The listing builds one solid part. Answer for the finished solid, in the listing's coordinates (mm). A direction names the side the tool comes from. Round coordinates to 2 decimals unless told otherwise and drop trailing zeros. Write each loop counter-clockwise with the first axis right and the second up, starting at its lowest first coordinate (ties: lowest second). Pieces come first, ordered by that corner, then holes.
Item 1: Find section D-D on y = 30. Give the vertices of the cut face in (x, z), then the cut area to 3 significant figures.
Item 2: Each of these flat-tipped pins is pushed along its axis until it touches: pin 1 (1 mm diameter, centred on y = 10, z = 1, fed in from +X); pin 2 (0.6 mm diameter, centred on y = -1, z = 1.5, fed in from +X). Where does it stop, or does it pass through?
Item 3: Find section C-C on x = 8. Give the vertices of the cut face in (y, z), then the cut area to 3 significant figures.
Item 4: Find section B-B on y = -1. Give the vertices of the cut face in (x, z), then the cut area to 3 significant figures.
Item 5: A tool of negligible diameter and unlimited length cuts with its end or side. For faces 1 (the face through (1, 32, 1)), 2 (the face through (3.877, -2, 1)), 3 (the face through (-3.877, 22, 1)), from which of +Z, -Z, +X, -X, +Y, -Y can it reach the whole face along a straight path? Write none if from no direction.
Item 6: Find the intervals of material crossed by probe 1 along Y at (x, z) = (0.5, 0.85); probe 2 along X at (y, z) = (18.5, 0.95); probe 3 along Y at (x, z) = (3.25, 1.35), in increasing order.
Item 7: For a pull along Y with two mould halves and no side action, classify faces 4 (the face through (0, 16, 1)), 5 (the face through (2.77, 2.71, 0.99)), 6 (the face through (-2.77, -2.71, 0.99)), 7 (the face through (9, 47, 1)) as +Y half, -Y half, draft (parallel to the pull), parting line (faces both ways), or undercut.
```python
from build123d import *

# Parameters (mm, degrees)
F0_R     = 1.875
F1_DEPTH = 2
F2_R     = 4.99999


# Not quite as in the source:
# - a fillet or chamfer is up to 0.001 mm smaller than in the source, because OpenCascade refuses the exact size


with BuildPart() as f1:
    # F0 (on Top) → F1 (new body)
    with BuildSketch(Plane.XY):
        with BuildLine():
            ThreePointArc((0, 3.876953125), (-2.741419845, 2.741419845), (-3.876953125, 0))
            ThreePointArc((-3.876953125, 0), (-2.741419845, -2.741419845), (0, -3.876953125))
            ThreePointArc((0, -3.876953125), (2.741419845, -2.741419845), (3.876953125, 0))
            ThreePointArc((3.876953125, 0), (2.741419845, 2.741419845), (0, 3.876953125))
        make_face()
        Circle(F0_R, mode=Mode.SUBTRACT)
        with BuildLine():
            Line((-3.876953125, 49), (-3.876953125, 0))
            ThreePointArc((-3.876953125, 0), (-2.741419845, 2.741419845), (0, 3.876953125))
            Line((0, 3.876953125), (0, 34))
            Line((0, 34), (10, 34))
            Line((10, 34), (10, 49))
            Line((10, 49), (-3.876953125, 49))
        make_face()
        with BuildLine():
            ThreePointArc((3.876953125, 0), (2.741419845, -2.741419845), (0, -3.876953125))
            Line((0, -3.876953125), (3.876953125, -3.876953125))
            Line((3.876953125, -3.876953125), (3.876953125, 0))
        make_face()
    extrude(amount=F1_DEPTH)

    # F2 (radius 5 in the source; OpenCascade refuses exactly that, so slightly less here)
    f2_edges = [f1.edges().sort_by_distance(p)[0] for p in [
        (0, 34, 1),
        (10, 34, 1),
        (10, 49, 1),
        (-3.876953, 49, 1),
    ]]
    fillet(f2_edges, radius=F2_R)


solid = f1.part
```
Check values:
1. outline: (-3.88, 0) - (0.1, 0) - (0.1, 2) - (-3.88, 2) - close
1. area: 7.96 mm2
2. pin 1: stops at x = 0
2. pin 2: stops at x = 3.88
3. outline: (35, 0) - (48, 0) - (48, 2) - (35, 2) - close
3. area: 26.0 mm2
4. outline: (-3.75, 0) - (-1.59, 0) - (-1.59, 2) - (-3.75, 2) - close; (1.59, 0) - (3.88, 0) - (3.88, 2) - (1.59, 2) - close
4. area: 8.90 mm2
5. face 1: +Z, -Z, +X
5. face 2: +Z, -Z, +X, -Y
5. face 3: +Z, -Z, -X, +Y, -Y
6. probe 1: y = -3.88 to -1.81, 1.81 to 3.84, 31.18 to 48.96
6. probe 2: x = -3.88 to 0
6. probe 3: y = -3.88 to 2.11, 33.68 to 49
7. face 4: undercut
7. face 5: undercut
7. face 6: -Y half
7. face 7: +Y half
